Check sheet for the modelled part. Datum: model origin and axes. Units: mm. A direction names the side the tool comes from. Round coordinates to 2 decimals unless told otherwise and drop trailing zeros. Order: outer loops, then holes, each group sorted by start corner. A loop starts at its lowest first (then second) coordinate and runs counter-clockwise, first axis right, second up.
Q1. Depth check by flat-ended pin: P1, Ø0.7, axis at x = 52.5, y = -5, coming from the +Z side; P2, Ø8, axis at x = 39, y = -23.5, coming from the -Z side; P3, Ø12, axis at x = 7.5, y = -6.5, coming from the -Z side. Enter the tip coordinate at first touch or a pass-through.
Q2. Cross-section at B-B on x = 10.5. Give the number of separate pieces and of enclosed holes in the cut face, then the cut area to 3 significant figures.
Q3. Set-up check for faces 1 (the flat face through (26, -14.211, 47)), 2 (the cylindrical face through (31.32, -19.47, 0.62)), 3 (the flat face through (26, -14.211, -46)): record each of +Z, -Z, +X, -X, +Y, -Y from which the full face is reachable in a straight line by a thin tool's end or side.
Q4. Scan lines: probe 1 along Z at (x, y) = (29.5, 0.5); probe 2 along Y at (x, z) = (22.5, 63.5); probe 3 along Y at (x, z) = (20, -26.5). Record each from-to range of solid material in increasing order.
Q5. Mould release check, pull along Z, two halves, no side actions. Record for faces 4 (the cylindrical face through (26.228, 0.312, 77.708)), 5 (the flat face through (0, -13, 0)), 6 (the flat face through (50.8, 0, 0)), 7 (the cylindrical face through (26.228, -0.312, -77.708)): +Z half, -Z half, draft (parallel to the pull), parting line (faces both ways), or undercut.
Q6. Cross-section at A-A on z = 0. Record the cut outline in (x, y).
Q7. Cross-section at C-C on z = -20. Record the cut outline in (x, y).
from build123d import *

# Parameters (mm, degrees)
SKETCH1_R           = 11.811
BOSS_EXTRUDE1_DEPTH = 50.8
BOSS_EXTRUDE2_DEPTH = 2.399999772
SKETCH4_W           = 53.199999772
SKETCH4_H           = 53.199999772
BOSS_EXTRUDE4_DEPTH = 12.7
CUT_EXTRUDE2_REACH  = 104.763
SKETCH5_R           = 4.7625
SKETCH7_W           = 53.199999772
SKETCH7_H           = 2.399999772
BOSS_EXTRUDE5_DEPTH = 23.622
CUT_EXTRUDE3_REACH  = 107.024
SKETCH10_W          = 2.794
SKETCH10_H          = 23.622
CUT_EXTRUDE4_DEPTH  = 2.54
FILLET1_R           = 2.54


with BuildPart() as part:
    # Sketch1 → Boss-Extrude1 (new body)
    with BuildSketch(Plane(origin=(0, 0, 0), x_dir=(0, 0, -1), z_dir=(1, 0, 0))):
        with BuildLine():
            Line((-63.5, 14.210999772), (63.5, 14.210999772))
            ThreePointArc((63.5, 14.210999772), (77.710999772, 0), (63.5, -14.210999772))
            Line((63.5, -14.210999772), (-63.5, -14.210999772))
            ThreePointArc((-63.5, -14.210999772), (-77.710999772, 0), (-63.5, 14.210999772))
        make_face()
        with Locations((-63.5, 0)):
            Circle(SKETCH1_R, mode=Mode.SUBTRACT)
        with Locations((63.5, 0)):
            Circle(SKETCH1_R, mode=Mode.SUBTRACT)
        with BuildLine():
            Line((-55.597292014, 11.811), (55.597292014, 11.811))
            ThreePointArc((55.597292014, 11.811), (49.289000228, 0), (55.597292014, -11.811))
            Line((55.597292014, -11.811), (-55.597292014, -11.811))
            ThreePointArc((-55.597292014, -11.811), (-49.289000228, 0), (-55.597292014, 11.811))
        make_face(mode=Mode.SUBTRACT)
    extrude(amount=BOSS_EXTRUDE1_DEPTH)

    # Sketch2 → Boss-Extrude2 (add)
    with BuildSketch(Plane(origin=(50.8, 0, 0), x_dir=(0, 0, -1), z_dir=(1, 0, 0))):
        with BuildLine():
            Line((-63.5, -14.210999772), (63.5, -14.210999772))
            ThreePointArc((63.5, -14.210999772), (77.710999772, 0), (63.5, 14.210999772))
            Line((63.5, 14.210999772), (-63.5, 14.210999772))
            ThreePointArc((-63.5, 14.210999772), (-77.710999772, 0), (-63.5, -14.210999772))
        make_face()
    extrude(amount=BOSS_EXTRUDE2_DEPTH)

    # Sketch4 → Boss-Extrude4 (add)
    with BuildSketch(Plane.XZ.offset(14.210999772)):
        with Locations((26.599999886, 0)):
            Rectangle(SKETCH4_W, SKETCH4_H)
    extrude(amount=BOSS_EXTRUDE4_DEPTH)

    # Sketch5 → Cut-Extrude2 (cut, up to next)
    with BuildSketch(Plane.XZ.offset(26.910999772), mode=Mode.PRIVATE) as cut_extrude2_sk1:
        with Locations(Location((26.599999886, 0, 0), (0, 0, 270))):
            Circle(SKETCH5_R)
    cut_extrude2_tool1 = extrude(cut_extrude2_sk1.sketch, amount=-CUT_EXTRUDE2_REACH, mode=Mode.PRIVATE) & part.part
    add(cut_extrude2_tool1.solids().sort_by_distance((26.6, -26.911, 0))[0], mode=Mode.SUBTRACT)

    # Sketch7 → Boss-Extrude5 (add)
    with BuildSketch(Plane(origin=(0, -11.811, 0), x_dir=(1, 0, 0), z_dir=(0, 1, 0))):
        with Locations((26.599999886, 7.549999886)):
            Rectangle(SKETCH7_W, SKETCH7_H)
        with Locations((26.599999886, -7.549999886)):
            Rectangle(SKETCH7_W, SKETCH7_H)
    extrude(amount=BOSS_EXTRUDE5_DEPTH)

    # Cut-Extrude3: up to this face of the body (flat: up to its plane)
    cut_extrude3_end = Plane(part.part.faces().sort_by_distance((25.4, 0, -8.749999772))[0])
    # Sketch9 → Cut-Extrude3 (cut, up to the picked face)
    with BuildSketch(Plane.XY.offset(8.749999772), mode=Mode.PRIVATE) as cut_extrude3_sk1:
        with BuildLine():
            Line((6.35, 3.175), (44.45, 3.175))
            ThreePointArc((44.45, 3.175), (47.625, 0), (44.45, -3.175))
            Line((44.45, -3.175), (6.35, -3.175))
            ThreePointArc((6.35, -3.175), (3.175, 0), (6.35, 3.175))
        make_face()
    cut_extrude3_tool1 = split(extrude(cut_extrude3_sk1.sketch, amount=-CUT_EXTRUDE3_REACH, mode=Mode.PRIVATE), bisect_by=cut_extrude3_end, keep=Keep.BOTH, mode=Mode.PRIVATE)
    add(cut_extrude3_tool1.solids().sort_by(Axis((25.4, 0, 8.75), (0, 0, -1)))[0], mode=Mode.SUBTRACT)

    # Sketch10 → Cut-Extrude4 (cut)
    with BuildSketch(Plane.ZY.offset(-50.8)):
        with Locations((-10.146999772, 0)):
            Rectangle(SKETCH10_W, SKETCH10_H)
        with Locations((10.146999772, 0)):
            Rectangle(SKETCH10_W, SKETCH10_H)
    extrude(amount=-CUT_EXTRUDE4_DEPTH, mode=Mode.SUBTRACT)

    # Fillet1
    fillet1_edges = [part.edges().sort_by_distance(p)[0] for p in [
        (26.599999886, -14.210999772, 26.599999886),
        (26.599999886, -14.210999772, -26.599999886),
        (50.8, 11.811, 0),
        (50.8, -11.811, 0),
    ]]
    fillet(fillet1_edges, radius=FILLET1_R)


solid = part.part
Results found:
1. P1: stops at z = 76.93
1. P2: stops at z = -26.6
1. P3: stops at z = -77.7
2. separate pieces: 1
2. enclosed holes: 3
2. area: 1,710 mm2
3. face 1: +Z, +X, -X, -Y
3. face 2: -Y
3. face 3: -Z, +X, -X, -Y
4. probe 1: z = -77.7 to -75.3, -51.7 to -49.3, 49.3 to 51.7, 75.3 to 77.7
4. probe 2: y = -14.21 to -11.81, 11.81 to 14.21
4. probe 3: y = -26.91 to -11.81, 11.81 to 14.21
5. face 4: +Z half
5. face 5: draft
5. face 6: undercut
5. face 7: -Z half
6. outline: (0, -26.91) - (21.84, -26.91) - (21.84, -11.81) - (0, -11.81) - close; (0, 11.81) - (48.26, 11.81) arc R2.54 cw to (50.8, 9.27) - (50.8, -9.27) arc R2.54 cw to (48.26, -11.81) - (31.36, -11.81) - (31.36, -26.91) - (53.2, -26.91) - (53.2, 14.21) - (0, 14.21) - close
7. outline: (0, -26.91) - (53.2, -26.91) - (53.2, 14.21) - (0, 14.21) - (0, 11.81) - (50.8, 11.81) - (50.8, -11.81) - (0, -11.81) - close
